Here's the drawing with two shaded views (mm, measured from the low corner). I have some questions. A direction names the side the tool comes from. Round coordinates to 2 decimals unless told otherwise and drop trailing zeros. Order: outer loops, then holes, each group sorted by start corner. A loop starts at its lowest first (then second) coordinate and runs counter-clockwise, first axis right, second up.
Q1. For the marked faces 1, 2 and 3, which set-ups out of +Z, -Z, +X, -X, +Y, -Y let a thin tool reach every point of the face, with its end or its side?
Q2. If we section it at B-B (z = 14.75): Please give me the cut outline in (x, y).
Q3. If I drill on line 1 (X direction, y = 3, z = 62); line 2 (Z direction, x = 74, y = 71); line 3 (Y direction, x = 75.5, z = 48), over which ranges is the centre line in solid material (lowest first)?
Q4. If we section it at D-D (z = 52): Please give me the cut outline in (x, y).
Q5. If we section it at A-A (y = 49): Please give me the cut outline in (x, z), plus the area to 3 significant figures.
Q6. If we section it at C-C (y = 71.5): Please give me the cut outline in (x, z), plus the area to 3 significant figures.
Q7. Will these pins go through, and if not, where does the flat tip stop? P1, Ø6.5, axis at y = 49, z = 47.47, coming from the -X side; P2, Ø3, axis at x = 98.5, z = 26.5, coming from the +Y side; P3, Ø1.5, axis at y = 94, z = 8.5, coming from the +X side.
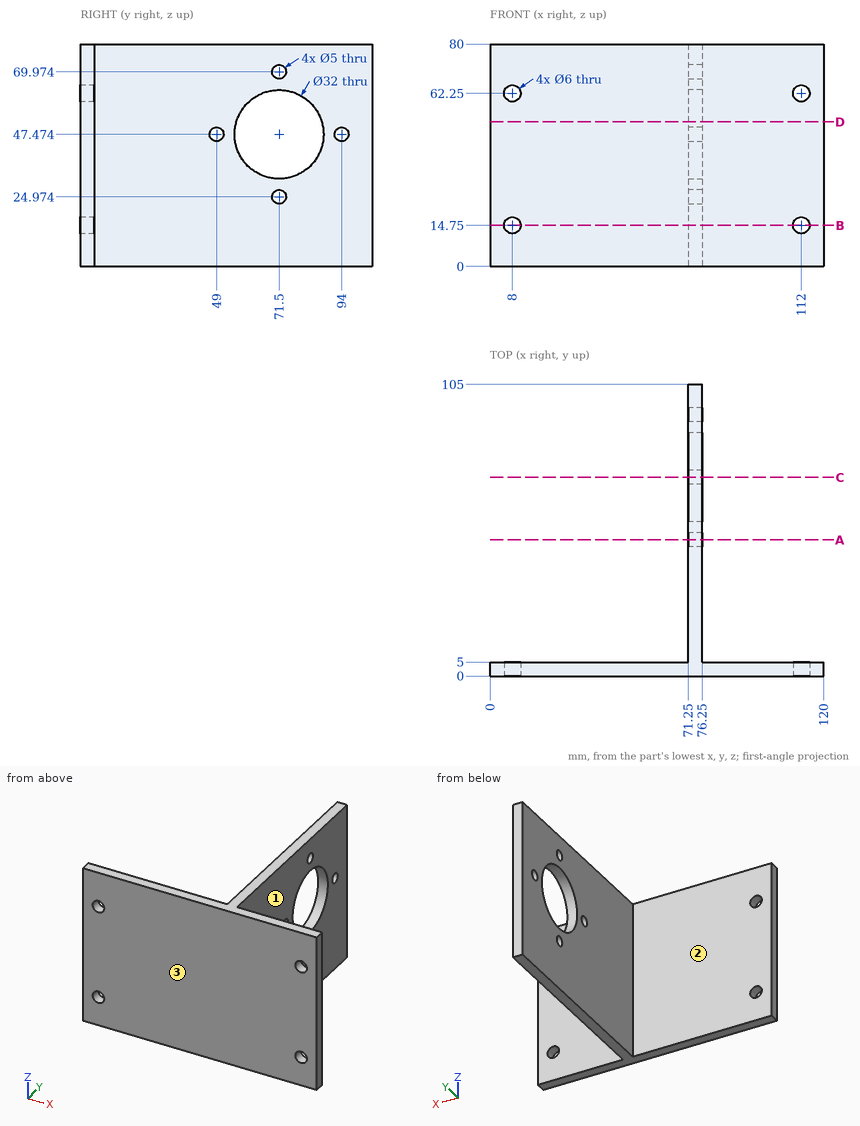
Solution:
1. face 1: +Z, -Z, +X, +Y
1. face 2: +Z, -Z, -X, +Y
1. face 3: +Z, -Z, +X, -X, -Y
2. outline: (0, 0) - (5, 0) - (5, 5) - (0, 5) - close; (11, 0) - (109, 0) - (109, 5) - (76.25, 5) - (76.25, 105) - (71.25, 105) - (71.25, 5) - (11, 5) - close; (115, 0) - (120, 0) - (120, 5) - (115, 5) - close
3. line 1: x = 0 to 5.01, 10.99 to 109.01, 114.99 to 120
3. line 2: z = 0 to 22.52, 27.42 to 31.48, 63.47 to 67.52, 72.42 to 80
3. line 3: y = 0 to 46.56, 51.44 to 55.51, 87.49 to 91.56, 96.44 to 105
4. outline: (0, 0) - (120, 0) - (120, 5) - (76.25, 5) - (76.25, 56.15) - (71.25, 56.15) - (71.25, 5) - (0, 5) - close; (71.25, 86.85) - (76.25, 86.85) - (76.25, 105) - (71.25, 105) - close
5. outline: (71.25, 0) - (76.25, 0) - (76.25, 44.97) - (71.25, 44.97) - close; (71.25, 49.97) - (76.25, 49.97) - (76.25, 80) - (71.25, 80) - close
5. area: 375 mm2
6. outline: (71.25, 0) - (76.25, 0) - (76.25, 22.47) - (71.25, 22.47) - close; (71.25, 27.47) - (76.25, 27.47) - (76.25, 31.47) - (71.25, 31.47) - close; (71.25, 63.47) - (76.25, 63.47) - (76.25, 67.47) - (71.25, 67.47) - close; (71.25, 72.47) - (76.25, 72.47) - (76.25, 80) - (71.25, 80) - close
6. area: 190 mm2
7. P1: stops at x = 71.25
7. P2: stops at y = 5
7. P3: stops at x = 76.25
